from build123d import *

# Parameters (mm, degrees)
F0_R     = 7.14375
F1_DEPTH = 1.8796


with BuildPart() as f1:
    # F0 (on Top) → F1 (new body)
    with BuildSketch(Plane.XY):
        with BuildLine():
            Line((0, 28.575), (0, 26.827432))
            ThreePointArc((0, 26.827432), (17.4625, 10.216869), (34.925, 26.827432))
            Line((34.925, 26.827432), (34.925, 28.575))
            Line((34.925, 28.575), (34.925, 914.4))
            Line((34.925, 914.4), (0, 914.4))
            Line((0, 914.4), (0, 28.575))
        make_face()
        with Locations((17.4625, 28.575)):
            Circle(F0_R, mode=Mode.SUBTRACT)
        with Locations((17.4625, 76.2)):
            Circle(F0_R, mode=Mode.SUBTRACT)
        with Locations((17.4625, 123.825)):
            Circle(F0_R, mode=Mode.SUBTRACT)
        with Locations((17.4625, 171.45)):
            Circle(F0_R, mode=Mode.SUBTRACT)
        with Locations((17.4625, 219.075)):
            Circle(F0_R, mode=Mode.SUBTRACT)
        with Locations((17.4625, 266.7)):
            Circle(F0_R, mode=Mode.SUBTRACT)
        with Locations((17.4625, 314.325)):
            Circle(F0_R, mode=Mode.SUBTRACT)
        with Locations((17.4625, 361.95)):
            Circle(F0_R, mode=Mode.SUBTRACT)
        with Locations((17.4625, 409.575)):
            Circle(F0_R, mode=Mode.SUBTRACT)
        with Locations((17.4625, 457.2)):
            Circle(F0_R, mode=Mode.SUBTRACT)
        with Locations((17.4625, 504.825)):
            Circle(F0_R, mode=Mode.SUBTRACT)
        with Locations((17.4625, 552.45)):
            Circle(F0_R, mode=Mode.SUBTRACT)
        with Locations((17.4625, 600.075)):
            Circle(F0_R, mode=Mode.SUBTRACT)
        with Locations((17.4625, 647.7)):
            Circle(F0_R, mode=Mode.SUBTRACT)
        with Locations((17.4625, 695.325)):
            Circle(F0_R, mode=Mode.SUBTRACT)
        with Locations((17.4625, 742.95)):
            Circle(F0_R, mode=Mode.SUBTRACT)
        with Locations((17.4625, 790.575)):
            Circle(F0_R, mode=Mode.SUBTRACT)
        with Locations((17.4625, 838.2)):
            Circle(F0_R, mode=Mode.SUBTRACT)
        with Locations((17.4625, 885.825)):
            Circle(F0_R, mode=Mode.SUBTRACT)
    extrude(amount=F1_DEPTH)


solid = f1.part
Geometry: final body of the model. Coordinates: model frame, mm. Coordinates: 2 decimals unless noted, no trailing zeros.
(1) Section query A-A (z = 0.7). State how many separate pieces and enclosed holes the cut face has, plus the area to 3 significant figures.
(2) First-contact query: pin 1 (8.5 mm diameter, centred on x = 17.46, y = 457.2, fed in from +Z) (3 decimals). Flat tip, straight axial feed; report the tip coordinate or a pass-through.
(3) Material intervals for probe 1 along X at (y, z) = (457.2, 0.6) (3 decimals); probe 2 along Y at (x, z) = (9, 0.1); probe 3 along Y at (x, z) = (9.5, 0.55), sorted ascending.
(4) Draft query along Y for faces 1 (the face through (17.09, 10.22, 0.93)), 2 (the face through (20.76, 879.49, 0.93)), 3 (the face through (17, 469, 0)). Return one class per face: pulls with the +Y half, pulls with the -Y half, needs draft (parallel to the pull), parting line crosses it, or undercut.
Solution:
1. separate pieces: 1
1. enclosed holes: 19
1. area: 28,400 mm2
2. pin 1: passes through
3. probe 1: x = 0 to 10.319, 24.606 to 34.925
3. probe 2: y = 12.4 to 914.4
3. probe 3: y = 12.14 to 914.4
4. face 1: pulls with the -Y half
4. face 2: undercut
4. face 3: needs draft
